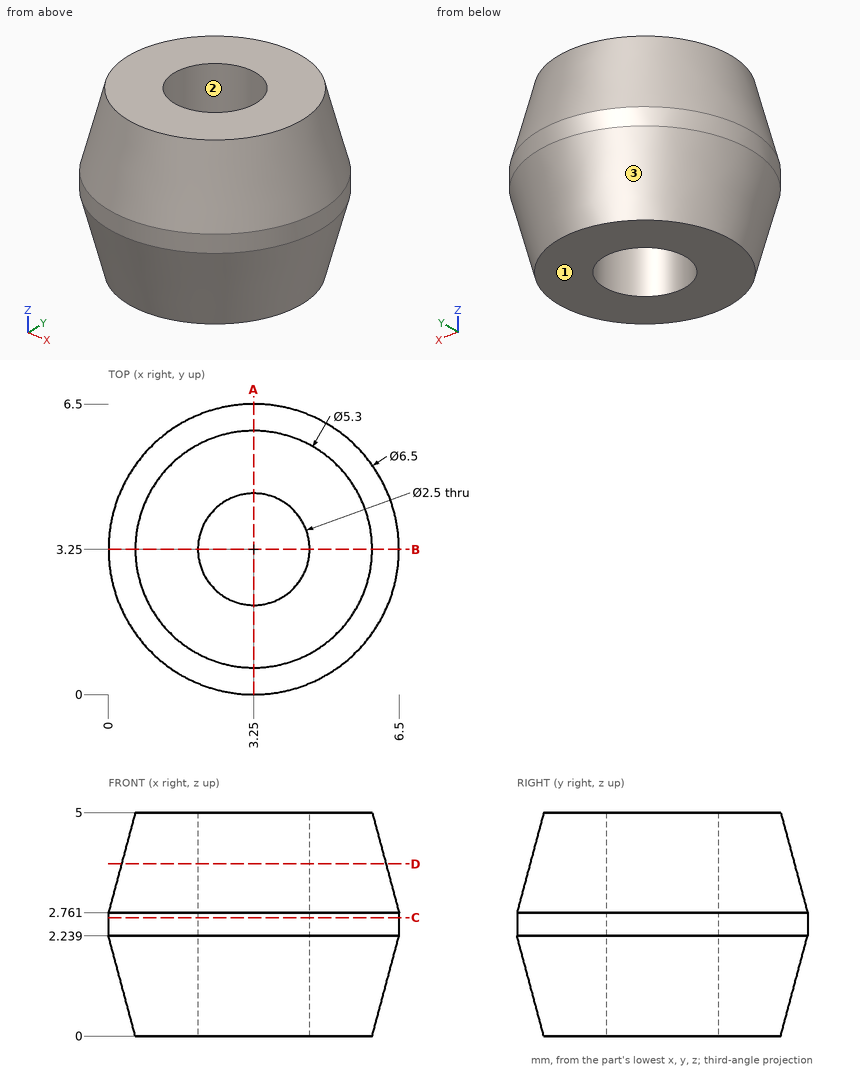
Could you check a few things on this drawing? It's one solid part, dimensions in mm from its lowest x, y, z. Coordinates: 2 decimals unless noted, no trailing zeros. Order: outer loops, then holes, each group sorted by start corner. A loop starts at its lowest first (then second) coordinate and runs counter-clockwise, first axis right, second up. Notation, with made-up numbers: (-27.5, 0) - (20.5, 0) arc R23 cw to (20.5, 27) - close; hole circle Ø6 at (86.25, -12.75). An arc over 180 degrees is marked (long way). One line per question, with ' | ' between items.
(1) Suppose I cut it at C-C on z = 2.65. List the corners of the cut face in (x, y) for me.
Report:
outline: circle Ø6.5 at (3.25, 3.25); hole circle Ø2.5 at (3.25, 3.25)
(2) If I drill on L1, parallel to Y at x = 3.25, z = 2.75; L2, parallel to X at y = 4, z = 0.35; L3, parallel to Y at x = 2.25, z = 2.2, over which ranges is the centre line in solid material (lowest first)?
Report:
L1: y = 0 to 2, 4.5 to 6.5 | L2: x = 0.61 to 2.25, 4.25 to 5.89 | L3: y = 0.17 to 2.5, 4 to 6.33
(3) Suppose I cut it at D-D on z = 3.85. List the corners of the cut face in (x, y) for me, and give its area (3 significant figures).
Report:
outline: circle Ø5.92 at (3.25, 3.25); hole circle Ø2.5 at (3.25, 3.25) | area: 22.6 mm2
(4) If we mould it in two halves opening along Y, with no side actions, what happens to the marked faces 1, 2 and 3? For each: pulls with the +Y half, pulls with the -Y half, needs draft (parallel to the pull), parting line crosses it, or undercut.
Report:
face 1: needs draft | face 2: undercut | face 3: parting line crosses it
(5) Suppose I cut it at A-A on x = 3.25. List the corners of the cut face in (y, z) for me.
Report:
outline: (0, 2.24) - (0.6, 0) - (2, 0) - (2, 5) - (0.6, 5) - (0, 2.76) - close; (4.5, 0) - (5.9, 0) - (6.5, 2.24) - (6.5, 2.76) - (5.9, 5) - (4.5, 5) - close
(6) Will these pins go through, and if not, where does the flat tip stop? pin 1 (3 mm diameter, centred on y = 1, z = 1.5, fed in from -X); pin 2 (2 mm diameter, centred on x = 3.25, y = 3.25, fed in from -Z); pin 3 (2 mm diameter, centred on x = 1, z = 1.5, fed in from +Y).
Report:
pin 1: stops at x = 0.14 | pin 2: passes through | pin 3: stops at y = 6.12
